```python
from build123d import *

# Parameters (mm, degrees)
SCHIZZO2_W                   = 62
SCHIZZO2_H                   = 50
ESTRUSIONE_ESTRUSIONE1_DEPTH = 3
FORO_PER_VITE_M3_1_D         = 3.4
SCHIZZO5_W                   = 42
SCHIZZO5_H                   = 8
TAGLIO_ESTRUSIONE1_DEPTH     = 3
SCHIZZO6_W                   = 45
SCHIZZO6_H                   = 26
TAGLIO_ESTRUSIONE2_DEPTH     = 3
RACCORDO1_R                  = 10
RACCORDO2_R                  = 4


with BuildPart() as part:
    # Schizzo2 → Estrusione-Estrusione1 (new body)
    with BuildSketch(Plane.XY):
        Rectangle(SCHIZZO2_W, SCHIZZO2_H)
    extrude(amount=ESTRUSIONE_ESTRUSIONE1_DEPTH)

    # Foro per Vite M3-1 (through all)
    with Locations(Plane.XY.offset(3)):
        with Locations((-26.586432577, -20), (26.586432577, -20)):
            Hole(FORO_PER_VITE_M3_1_D / 2)

    # Schizzo5 → Taglio-Estrusione1 (cut)
    with BuildSketch(Plane.XY.offset(3)):
        with Locations((0, -21)):
            Rectangle(SCHIZZO5_W, SCHIZZO5_H)
    extrude(amount=-TAGLIO_ESTRUSIONE1_DEPTH, mode=Mode.SUBTRACT)

    # Schizzo6 → Taglio-Estrusione2 (cut)
    with BuildSketch(Plane.XY.offset(3)):
        with Locations((0, 3.772071737)):
            Rectangle(SCHIZZO6_W, SCHIZZO6_H)
    extrude(amount=-TAGLIO_ESTRUSIONE2_DEPTH, mode=Mode.SUBTRACT)

    # Raccordo1
    raccordo1_edges = [part.edges().sort_by_distance(p)[0] for p in [
        (-31, 25, 1.5),
        (31, 25, 1.5),
    ]]
    fillet(raccordo1_edges, radius=RACCORDO1_R)

    # Raccordo2
    raccordo2_edges = [part.edges().sort_by_distance(p)[0] for p in [
        (-21, -25, 1.5),
        (21, -25, 1.5),
        (31, -25, 1.5),
        (-31, -25, 1.5),
    ]]
    fillet(raccordo2_edges, radius=RACCORDO2_R)


solid = part.part
```
Read the model definition and answer for the solid it produces. Units are mm, in the model's axes. A direction names the side the tool comes from. Round coordinates to 2 decimals unless told otherwise and drop trailing zeros. Loops run counter-clockwise (first coordinate to the right, second up) from the corner with the lowest first, then second, coordinate; pieces in that order, holes last. Notation, with made-up numbers: (18.5, 10) -> (44.5, 10) arc R20 ccw to (44.5, 24) -> close; hole circle Ø5 at (-17, 42.25). An arc over 180 degrees is marked (long way). One line per item, written item: value.
1) For faces 4 (the face through (-21, -19, 2)), 5 (the face through (-26, -25, 1)), 6 (the face through (22.5, 4, 2)), determine the directions among +Z, -Z, +X, -X, +Y, -Y from which every point of the face is accessible in a straight line to the end or side of a thin tool.
Answer list:
face 4: +Z, -Z, -Y
face 5: +Z, -Z, +X, -X, -Y
face 6: +Z, -Z
2) A cutting plane is placed at A-A (y = -20). Determine the outline of the cut face in (x, z), and give its area (3 significant figures).
Answer list:
outline: (-31, 0) -> (-28.29, 0) -> (-28.29, 3) -> (-31, 3) -> close; (-24.89, 0) -> (-21, 0) -> (-21, 3) -> (-24.89, 3) -> close; (21, 0) -> (24.89, 0) -> (24.89, 3) -> (21, 3) -> close; (28.29, 0) -> (31, 0) -> (31, 3) -> (28.29, 3) -> close
area: 39.6 mm²
3) Consider L1, parallel to X at y = -5.5, z = 1.55; L2, parallel to Y at x = -10, z = 0.2; L3, parallel to X at y = -22, z = 2.2. Determine where each line is inside the solid, lowest interval first. Write a range as [from, to].
Answer list:
L1: x = [-31, -22.5], [22.5, 31]
L2: y = [-17, -9.23], [16.77, 25]
L3: x = [-30.87, -21.13], [21.13, 30.87]
4) The mould has two halves that part along Y. Classify faces 1 (the face through (-28.21, -19.49, 1.48)), 2 (the face through (31, -3, 1)), 3 (the face through (-22.203, -23.859, 1.479)): pulls with the +Y half, pulls with the -Y half, needs draft (parallel to the pull), parting line crosses it, or undercut.
Answer list:
face 1: undercut
face 2: needs draft
face 3: pulls with the -Y half
5) A flat-ended cylindrical pin translates along its axis: P1, Ø0.9, axis at x = 7.5, z = 1.5, coming from the -Y side. Find the tip coordinate at first contact, or state that the pin passes through.
Answer list:
P1: stops at y = -17
6) A cutting plane is placed at C-C (z = 2.05). Determine the outline of the cut face in (x, y), and give its area (3 significant figures).
Answer list:
outline: (-31, -21) arc R4 ccw to (-27, -25) -> (-25, -25) arc R4 ccw to (-21, -21) -> (-21, -17) -> (21, -17) -> (21, -21) arc R4 ccw to (25, -25) -> (27, -25) arc R4 ccw to (31, -21) -> (31, 15) arc R10 ccw to (21, 25) -> (-21, 25) arc R10 ccw to (-31, 15) -> close; hole circle Ø3.4 at (-26.59, -20); hole (-22.5, -9.23) -> (22.5, -9.23) -> (22.5, 16.77) -> (-22.5, 16.77) -> close; hole circle Ø3.4 at (26.59, -20)
area: 1,520 mm²
7) A cutting plane is placed at B-B (x = 20). Determine the outline of the cut face in (y, z).
Answer list:
outline: (-17, 0) -> (-9.23, 0) -> (-9.23, 3) -> (-17, 3) -> close; (16.77, 0) -> (25, 0) -> (25, 3) -> (16.77, 3) -> close
